The listing builds one solid part. Answer for the finished solid, in the listing's coordinates (mm). A direction names the side the tool comes from. Coordinates: 2 decimals unless noted, no trailing zeros. Write each loop counter-clockwise with the first axis right and the second up, starting at its lowest first coordinate (ties: lowest second). Pieces come first, ordered by that corner, then holes.
```python
from build123d import *

# Parameters (mm, degrees)
SKETCH_2_W          = 55
SKETCH_2_H          = 90
EXTRUDE_1_DEPTH     = 10
FILLET_1_R          = 5
FILLET_2_R          = 5
FILLET_3_R          = 5
FILLET_4_R          = 5
SKETCH_3_W          = 5
SKETCH_3_H          = 10
CUT_EXTRUDE_1_DEPTH = 5


with BuildPart() as part:
    # 草图2 → 凸台-拉伸1 (new body)
    with BuildSketch(Plane(origin=(0, 0, 0), x_dir=(1, 0, 0), z_dir=(0, 1, 0))):
        Rectangle(SKETCH_2_W, SKETCH_2_H)
    extrude(amount=EXTRUDE_1_DEPTH)

    # 圆角1
    fillet_1_edges = [part.edges().sort_by_distance(p)[0] for p in [
        (-27.5, 10, 0),
    ]]
    fillet(fillet_1_edges, radius=FILLET_1_R)

    # 圆角2
    fillet_2_edges = [part.edges().sort_by_distance(p)[0] for p in [
        (-27.5, 2.5, -45),
        (-26.035533906, 8.535533906, -45),
        (2.5, 10, -45),
    ]]
    fillet(fillet_2_edges, radius=FILLET_2_R)

    # 圆角3
    fillet_3_edges = [part.edges().sort_by_distance(p)[0] for p in [
        (27.5, 2.5, -45),
        (27.5, 8.535533906, -43.535533906),
        (27.5, 10, 2.5),
    ]]
    fillet(fillet_3_edges, radius=FILLET_3_R)

    # 圆角4
    fillet_4_edges = [part.edges().sort_by_distance(p)[0] for p in [
        (0, 10, 45),
        (-27.5, 2.5, 45),
        (-26.035533906, 8.535533906, 45),
        (27.5, 2.5, 45),
        (26.035533906, 8.535533906, 45),
    ]]
    fillet(fillet_4_edges, radius=FILLET_4_R)

    # 草图3 → 切除-拉伸1 (cut)
    with BuildSketch(Plane(origin=(0, 10, 0), x_dir=(1, 0, 0), z_dir=(0, 1, 0))):
        with Locations((-19.5, 20)):
            Rectangle(SKETCH_3_W, SKETCH_3_H)
        with Locations((-19.5, -20)):
            Rectangle(SKETCH_3_W, SKETCH_3_H)
    extrude(amount=-CUT_EXTRUDE_1_DEPTH, mode=Mode.SUBTRACT)


solid = part.part
```
(1) Section B-B, the plane z = -19 is taken. Write down the section's boundary in (x, y).
(2) Find the intervals of material crossed by probe 1 along Y at (x, z) = (-20, -16); probe 2 along Z at (x, y) = (-21.5, 6); probe 3 along Z at (x, y) = (-18, 8.25), in increasing order.
(3) Section A-A, the plane y = 8 is taken. Write down the section's boundary in (x, z), plus the area to 3 significant figures.
(4) Which of the six approach directions +Z, -Z, +X, -X, +Y, -Y give full straight-line access (tool end or side, diameter ignored) to faces 1 (the flat face through (-20, 8, -25)), 2 (the flat face through (0, 0, -1))?
(5) For a pull along Z with two mould halves and no side action, classify faces 3 (the cylindrical face through (26, 2.54, -43.57)), 4 (the cylindrical face through (-26, 2.54, 43.57)), 5 (the flat face through (-20, 8, -15)), 6 (the flat face through (-20, 8, 25)) as pulls with the +Z half, pulls with the -Z half, needs draft (parallel to the pull), parting line crosses it, or undercut.
(6) Each of these flat-tipped pins is pushed along its axis until it touches: pin 1 (1.5 mm diameter, centred on x = -20.5, y = 8.5, fed in from -Z); pin 2 (2.5 mm diameter, centred on x = -19, y = 8.5, fed in from +Z); pin 3 (1.5 mm diameter, centred on y = 6.5, z = 18, fed in from -X). Where does it stop, or does it pass through?
Solution:
1. outline: (-27.5, 0) - (27.5, 0) - (27.5, 5) arc R5 ccw to (22.5, 10) - (-17, 10) - (-17, 5) - (-22, 5) - (-22, 10) - (-22.5, 10) arc R5 ccw to (-27.5, 5) - close
2. probe 1: y = 0 to 5
2. probe 2: z = -44.9 to -25, -15 to 15, 25 to 44.9
2. probe 3: z = -43.8 to -25, -15 to 15, 25 to 43.8
3. outline: (-26.5, -40) arc R4 ccw to (-22.5, -44) - (22.5, -44) arc R4 ccw to (26.5, -40) - (26.5, 40) arc R4 ccw to (22.5, 44) - (-22.5, 44) arc R4 ccw to (-26.5, 40) - close; hole (-22, -25) - (-17, -25) - (-17, -15) - (-22, -15) - close; hole (-22, 15) - (-17, 15) - (-17, 25) - (-22, 25) - close
3. area: 4,550 mm2
4. face 1: +Y
4. face 2: +Z, -Z, +X, -X, -Y
5. face 3: pulls with the -Z half
5. face 4: pulls with the +Z half
5. face 5: undercut
5. face 6: undercut
6. pin 1: stops at z = -44.18
6. pin 2: stops at z = 44.47
6. pin 3: stops at x = -27.44
